The model under review builds one solid part; all positions refer to its coordinate system, in mm. Round coordinates to 2 decimals unless told otherwise and drop trailing zeros. Write each loop counter-clockwise with the first axis right and the second up, starting at its lowest first coordinate (ties: lowest second). Pieces come first, ordered by that corner, then holes. Notation, with made-up numbers: (43.5, 34.5) -> (75.5, 34.5) arc R4 cw to (75.5, 38.5) -> close; hole circle Ø2 at (32.25, 51.5). An arc over 180 degrees is marked (long way). Answer as a JSON object with one key per item and string values. Group by question number.
1) Mouldability with a two-part tool opening along Y and no side actions: class faces 1 (the flat face through (-12, 28, 150)), 2 (the cylindrical face through (-29.97, 1.32, 2.1)), 3 (the cylindrical face through (-30.97, -1.36, -2.1)) as pulls with the +Y half, pulls with the -Y half, needs draft (parallel to the pull), parting line crosses it, or undercut.
2) We need section C-C, the plane z = 46. Write out the cut boundary in (x, y), then the cut area to 3 significant figures.
3) We need section D-D, the plane x = -18. Write out the cut boundary in (y, z), then the cut area to 3 significant figures.
4) We need section A-A, the plane x = 0. Write out the cut boundary in (y, z), then the cut area to 3 significant figures.
5) Insertion check: pin 1 Ø1.5 at (y, z) = (16, 24.5) entering from +X; pin 2 Ø1.2 at (y, z) = (-28.5, 20) entering from +X; pin 3 Ø4 at (x, z) = (7.5, -19.5) entering from +Y. Each pin has a flat end and moves straight along its axis. Give the tip position at first contact, or say it passes through.
6) We need section B-B, the plane y = -8.5. Count the separate pieces of the cut face and the enclosed holes in it, then the cut area to 3 significant figures.
7) To check wall thickness, follow probe 1 along Y at (x, z) = (0, -40); probe 2 along Y at (x, z) = (7.5, -42); probe 3 along X at (y, z) = (1, -102). State the ranges of each line that lie inside material, in increasing order. Write a range as [from, to].
Autodesk Inventor part; units mm, degrees
ref_plane "YZ Plane" through (0, 0, 0) normal (1, 0, 0) x (0, 1, 0)
ref_plane "XZ Plane" through (0, 0, 0) normal (0, 1, 0) x (-1, 0, 0)
ref_plane "XY Plane" through (0, 0, 0) normal (0, 0, 1) x (1, 0, 0)
sketch "Skizze1" plane through (0, 0, 0) normal (0, 0, 1) x (1, 0, 0)
  circle A0 centre (0, 0) radius 31
  circle A1 centre (0, 0) radius 30
  dimension "d0" = 62
  dimension "d1" = 60
extrude "Extrusion1" add sketch "Skizze1" along normal mid plane 300
sketch "Skizze2" plane through (0, 0, 0) normal (0, 1, 0) x (-1, 0, 0)
  line L0 (-10, 169.5773) -> (-10, -169.8146) construction
  line L1 (-74.8376, 0) -> (82.6362, 0) construction
  line L2 (-10, 75) -> (-10, -75)
  line L3 (-31, -150) -> (-31, 150)
  line L4 (31, 150) -> (-31, 150)
  line L5 (-31, -150) -> (31, -150)
  spline S0 degree 2 poles (-10, 75) (-18.1599, 136.3675) (-72.8449, 128.3193) knots 0 0 0 1 1 1
  spline S1 degree 2 poles (-10, -75) (-17.9565, -136.1553) (-74.8376, -130) knots 0 0 0 1 1 1
  line L6 (-72.8449, 128.3193) -> (-74.8376, -130)
  point P0 (0, 0)
  point P1 (-31, 120)
  point P2 (-31, -120)
  dimension "d4" = 10
  dimension "d5" = 150
  dimension "d6" = 30
  dimension "d7" = 30
extrude "Extrusion2" cut sketch "Skizze2" against normal mid plane 65 contours L2 S1 L3 S0
properties part number "Segment_mitte"
Here are the results:
{
 "1": {"face 1": "needs draft", "face 2": "undercut", "face 3": "parting line crosses it"},
 "2": {"outline": "(10, -29.34) -> (10, -28.28) arc R30 cw (long way) to (10, 28.28) -> (10, 29.34) arc R31 ccw (long way) to start", "area": "116 mm^2"},
 "3": {"outline": "(-25.24, -150) -> (-24, -150) -> (-24, 150) -> (-25.24, 150) -> close; (24, -150) -> (25.24, -150) -> (25.24, 150) -> (24, 150) -> close", "area": "743 mm^2"},
 "4": {"outline": "(-31, -150) -> (-30, -150) -> (-30, 150) -> (-31, 150) -> close; (30, -150) -> (31, -150) -> (31, 150) -> (30, 150) -> close", "area": "600 mm^2"},
 "5": {"pin 1": "stops at x = -24.89", "pin 2": "stops at x = 10", "pin 3": "stops at y = 30.51"},
 "6": {"separate pieces": "3", "enclosed holes": "0", "area": "378 mm^2"},
 "7": {"probe 1": "y = [-31, -30], [30, 31]", "probe 2": "y = [-30.08, -29.05], [29.05, 30.08]", "probe 3": "x = [-30.98, -29.98]"}
}
